Geometry check sheet. Reference: the model listing, model coordinates, mm. Face numbers are marked on the shaded views. Round coordinates to 2 decimals unless told otherwise and drop trailing zeros. Write each loop counter-clockwise with the first axis right and the second up, starting at its lowest first coordinate (ties: lowest second). Pieces come first, ordered by that corner, then holes. Notation, with made-up numbers: M 26,63 L 85,63 A22 ccw 85,75 Z; hole C -32.5,25.5 d6. An arc over 180 degrees is marked long. Put each result on its own line as item: value. Start each with the question number.
(1) Section check A-A on z = -13. Count the separate pieces of the cut face and the enclosed holes in it, then the cut area to 3 significant figures.
(2) Mould release check, pull along Z, two halves, no side actions. Record for the marked faces 1 and 2: pulls with the +Z half, pulls with the -Z half, needs draft (parallel to the pull), parting line crosses it, or undercut.
(3) Section check B-B on x = 26.5. Record the cut outline in (y, z) (3 decimals), then the cut area to 3 significant figures.
(4) Material ranges on probe 1 along Z at (x, y) = (5, 1.6); probe 2 along Z at (x, y) = (16, 0.45) (3 decimals); probe 3 along Z at (x, y) = (35, 3.05), recorded low to high.
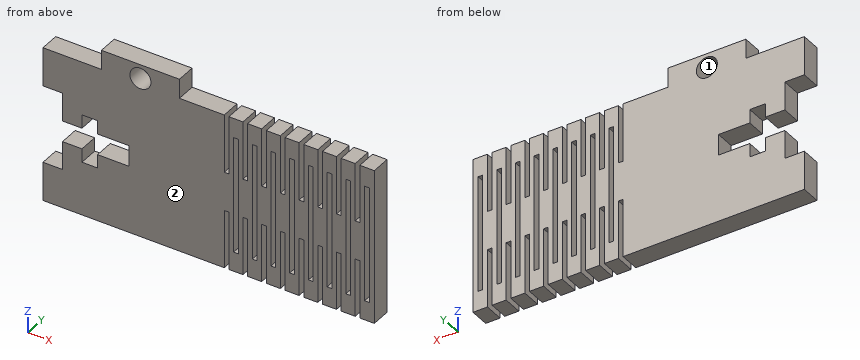
from build123d import *

# Parameters (mm, degrees)
SKETCH1_R           = 1.7145
BOSS_EXTRUDE1_DEPTH = 3.175
SKETCH3_W           = 25.4
SKETCH3_H           = 3.175
BOSS_EXTRUDE2_DEPTH = 25.4
SKETCH4_W           = 0.762
SKETCH4_H           = 9.525
SKETCH4_H_2         = 19.05
CUT_EXTRUDE2_DEPTH  = 60.737268518


with BuildPart() as part:
    # Sketch1 → Boss-Extrude1 (new body)
    with BuildSketch(Plane(origin=(0, 0, 0), x_dir=(1, 0, 0), z_dir=(0, 1, 0))):
        Polygon((0, 19.05), (3.175, 19.05), (3.175, 14.4145), (6.35, 14.4145), (6.35, 16.637), (8.89, 16.637), (8.89, 14.4145), (13.97, 14.4145), (13.97, 10.9855), (8.89, 10.9855), (8.89, 8.763), (6.35, 8.763), (6.35, 10.9855), (3.175, 10.9855), (3.175, 6.35), (0, 6.35), (0, 0), (9.525, 0), (9.525, -3.175), (22.225, -3.175), (22.225, 0), (28.575, 0), (28.575, 25.4), (0, 25.4), align=None)
        with Locations(Location((15.875, -0.889, 0), (0, 0, 270))):
            Circle(SKETCH1_R, mode=Mode.SUBTRACT)
    extrude(amount=BOSS_EXTRUDE1_DEPTH)

    # Sketch3 → Boss-Extrude2 (add)
    with BuildSketch(Plane(origin=(28.575, 0, 0), x_dir=(0, 0, -1), z_dir=(1, 0, 0))):
        with Locations((12.7, 1.5875)):
            Rectangle(SKETCH3_W, SKETCH3_H)
    extrude(amount=BOSS_EXTRUDE2_DEPTH)

    # Sketch4 → Cut-Extrude2 (cut, through all)
    with BuildSketch(Plane(origin=(0, 3.175, 0), x_dir=(1, 0, 0), z_dir=(0, 1, 0))):
        with Locations((29.908251949, 4.7625)):
            Rectangle(SKETCH4_W, SKETCH4_H)
        with Locations((31.432251949, 12.7)):
            Rectangle(SKETCH4_W, SKETCH4_H_2)
        with Locations((29.908251949, 20.6375)):
            Rectangle(SKETCH4_W, SKETCH4_H)
        with Locations((32.956251949, 4.7625)):
            Rectangle(SKETCH4_W, SKETCH4_H)
        with Locations((34.480251949, 12.7)):
            Rectangle(SKETCH4_W, SKETCH4_H_2)
        with Locations((32.956251949, 20.6375)):
            Rectangle(SKETCH4_W, SKETCH4_H)
        with Locations((36.004251949, 4.7625)):
            Rectangle(SKETCH4_W, SKETCH4_H)
        with Locations((37.528251949, 12.7)):
            Rectangle(SKETCH4_W, SKETCH4_H_2)
        with Locations((36.004251949, 20.6375)):
            Rectangle(SKETCH4_W, SKETCH4_H)
        with Locations((39.052251949, 4.7625)):
            Rectangle(SKETCH4_W, SKETCH4_H)
        with Locations((40.576251949, 12.7)):
            Rectangle(SKETCH4_W, SKETCH4_H_2)
        with Locations((39.052251949, 20.6375)):
            Rectangle(SKETCH4_W, SKETCH4_H)
        with Locations((42.100251949, 4.7625)):
            Rectangle(SKETCH4_W, SKETCH4_H)
        with Locations((43.624251949, 12.7)):
            Rectangle(SKETCH4_W, SKETCH4_H_2)
        with Locations((42.100251949, 20.6375)):
            Rectangle(SKETCH4_W, SKETCH4_H)
        with Locations((45.148251949, 4.7625)):
            Rectangle(SKETCH4_W, SKETCH4_H)
        with Locations((46.672251949, 12.7)):
            Rectangle(SKETCH4_W, SKETCH4_H_2)
        with Locations((45.148251949, 20.6375)):
            Rectangle(SKETCH4_W, SKETCH4_H)
        with Locations((48.196251949, 4.7625)):
            Rectangle(SKETCH4_W, SKETCH4_H)
        with Locations((49.720251949, 12.7)):
            Rectangle(SKETCH4_W, SKETCH4_H_2)
        with Locations((48.196251949, 20.6375)):
            Rectangle(SKETCH4_W, SKETCH4_H)
        with Locations((51.244251949, 4.7625)):
            Rectangle(SKETCH4_W, SKETCH4_H)
        with Locations((52.768251949, 12.7)):
            Rectangle(SKETCH4_W, SKETCH4_H_2)
        with Locations((51.244251949, 20.6375)):
            Rectangle(SKETCH4_W, SKETCH4_H)
    extrude(amount=-CUT_EXTRUDE2_DEPTH, mode=Mode.SUBTRACT)


solid = part.part
Answers follow:
1. separate pieces: 9
1. enclosed holes: 0
1. area: 108 mm^2
2. face 1: undercut
2. face 2: needs draft
3. outline: M 0,-25.4 L 3.175,-25.4 L 3.175,0 L 0,0 Z
3. area: 80.6 mm^2
4. probe 1: z = -25.4 to -14.41, -10.99 to 0
4. probe 2: z = -25.4 to -0.821, 2.599 to 3.175
4. probe 3: z = -25.4 to 0
